Geometry check sheet. Reference: the model listing, model coordinates, mm. A direction names the side the tool comes from. Give positions to 0.01 mm unless a question says otherwise; leave off trailing zeros. Order: outer loops, then holes, each group sorted by start corner. A loop starts at its lowest first (then second) coordinate and runs counter-clockwise, first axis right, second up. Notation, with made-up numbers: M 71,78 L 79,78 A35 ccw 79,115 Z; hole C 18,8.25 d6. An arc over 180 degrees is marked long. Answer as a JSON object with one key per item and string values. Group by question number.
from build123d import *

# Parameters (mm, degrees)
F1_DEPTH     = 2
F3_DEPTH     = 13
F4_DEPTH     = 11
F5_R         = 1.5
F6_DEPTH     = 8
F7_T4_DEPTH  = 97.0812194284
F7_T9_DEPTH  = 97.0812194284
F7_T14_DEPTH = 97.0812194284
F7_T20_DEPTH = 97.0812194284
F7_T25_DEPTH = 97.0812194284
F7_T31_DEPTH = 97.0812194284
F8_R         = 1


# Not quite as in the source:
# - a fillet or chamfer that OpenCascade refuses, or shapes differently, is made with other operations: its cross-section is extruded or revolved along the edge and cut away or added


with BuildPart() as f1:
    # F0 (on Top) → F1 (new body)
    with BuildSketch(Plane.XY):
        Polygon((0, 9.3), (0, 0), (67, 0), (67, 6), align=None)
    extrude(amount=F1_DEPTH)

    # F2 (on face) → F3 (join)
    with BuildSketch(Plane.XY.offset(2)):
        Polygon((0.7854075007, 8.5), (0.7854075007, 0.5), (8.7757214003, 8.1064472258), align=None)
    extrude(amount=-F3_DEPTH)

    # F2 (on face) → F4 (join)
    with BuildSketch(Plane.XY.offset(2)):
        Polygon((62.9, 1.65), (66.9, 5.8), (53.9157399132, 6.439523258), (57.3, 1.65), align=None)
    extrude(amount=-F4_DEPTH)

    # F5 (on face) → F6 (cut)
    with BuildSketch(Plane(origin=(0, 0, -11), x_dir=(1, 0, 0), z_dir=(0, 0, -1))):
        with Locations((3.1854075007, -5.9788816921)):
            Circle(F5_R)
        with Locations((60.0157399132, -3.9364085902)):
            Circle(F5_R)
    extrude(amount=-F6_DEPTH, mode=Mode.SUBTRACT)

    # F7: fillet of radius 10 on 1 edges, made by hand


with BuildPart() as f7_tool2:
    # F7_s3 → F7_t4 (new body)
    with BuildSketch(Plane(origin=(81.5248873918, -4.0154049014, 0), x_dir=(0, 0, 1), z_dir=(-0.9987892374, 0.0491940968, 0))):
        with BuildLine():
            ThreePointArc((2, 9.2887399083), (0.5131670195, 6.4510175684), (0, 3.2887399083))
            Line((0, 3.2887399083), (0, 9.2887399083))
            Line((0, 9.2887399083), (2, 9.2887399083))
        make_face()
    extrude(amount=F7_T4_DEPTH)

    split(bisect_by=Plane(origin=(0.4468822571, 9.0730640082, 0), x_dir=(0, 0, 1), z_dir=(0.0491940968, 0.9987892374, 0)), keep=Keep.TOP)


with BuildPart() as f1_1:
    add(f1.part)

    # F7_t1: cut F7_tool2
    add(f7_tool2.part, mode=Mode.SUBTRACT)


with BuildPart() as f7_tool7:
    # F7_s8 → F7_t9 (new body)
    with BuildSketch(Plane(origin=(81.5248873918, -4.0154049014, 0), x_dir=(0, 0, 1), z_dir=(-0.9987892374, 0.0491940968, 0))):
        with BuildLine():
            ThreePointArc((2, 9.2887399083), (0.5131670195, 6.4510175684), (0, 3.2887399083))
            Line((0, 3.2887399083), (0, 9.2887399083))
            Line((0, 9.2887399083), (2, 9.2887399083))
        make_face()
    extrude(amount=F7_T9_DEPTH)

    split(bisect_by=Plane(origin=(31.7828354278, -30.6340582437, 0), x_dir=(0, 0, 1), z_dir=(0.7199990803, -0.6939750171, 0)), keep=Keep.TOP)


with BuildPart() as f1_2:
    add(f1_1.part)

    # F7_t6: cut F7_tool7
    add(f7_tool7.part, mode=Mode.SUBTRACT)


with BuildPart() as f7_tool12:
    # F7_s13 → F7_t14 (new body)
    with BuildSketch(Plane(origin=(81.5248873918, -4.0154049014, 0), x_dir=(0, 0, 1), z_dir=(-0.9987892374, 0.0491940968, 0))):
        with BuildLine():
            ThreePointArc((2, 9.2887399083), (0.5131670195, 6.4510175684), (0, 3.2887399083))
            Line((0, 3.2887399083), (0, 9.2887399083))
            Line((0, 9.2887399083), (2, 9.2887399083))
        make_face()
    extrude(amount=F7_T14_DEPTH)

    split(bisect_by=Plane(origin=(38.996012386, 27.554443554, 0), x_dir=(0, 0, 1), z_dir=(-0.816693011, -0.5770723748, 0)), keep=Keep.TOP)

    split(bisect_by=Plane(origin=(0.1236877347, -0.1299297552, 0), x_dir=(0, 0, 1), z_dir=(0.6894947075, -0.7242907209, 0)), keep=Keep.TOP)


with BuildPart() as f1_3:
    add(f1_2.part)

    # F7_t11: cut F7_tool12
    add(f7_tool12.part, mode=Mode.SUBTRACT)


with BuildPart() as f7_tool18:
    # F7_s19 → F7_t20 (new body)
    with BuildSketch(Plane(origin=(81.5248873918, -4.0154049014, 0), x_dir=(0, 0, 1), z_dir=(-0.9987892374, 0.0491940968, 0))):
        with BuildLine():
            ThreePointArc((2, 9.2887399083), (0.5131670195, 6.4510175684), (0, 3.2887399083))
            Line((0, 3.2887399083), (0, 9.2887399083))
            Line((0, 9.2887399083), (2, 9.2887399083))
        make_face()
    extrude(amount=F7_T20_DEPTH)

    split(bisect_by=Plane.XZ.offset(-1.65), keep=Keep.TOP)


with BuildPart() as f1_4:
    add(f1_3.part)

    # F7_t17: cut F7_tool18
    add(f7_tool18.part, mode=Mode.SUBTRACT)


with BuildPart() as f7_tool23:
    # F7_s24 → F7_t25 (new body)
    with BuildSketch(Plane(origin=(81.5248873918, -4.0154049014, 0), x_dir=(0, 0, 1), z_dir=(-0.9987892374, 0.0491940968, 0))):
        with BuildLine():
            ThreePointArc((2, 9.2887399083), (0.5131670195, 6.4510175684), (0, 3.2887399083))
            Line((0, 3.2887399083), (0, 9.2887399083))
            Line((0, 9.2887399083), (2, 9.2887399083))
        make_face()
    extrude(amount=F7_T25_DEPTH)

    split(bisect_by=Plane(origin=(0.419544275, 8.518020129, 0), x_dir=(0, 0, 1), z_dir=(0.0491940968, 0.9987892374, 0)), keep=Keep.TOP)

    split(bisect_by=Plane(origin=(0.1236877347, -0.1299297552, 0), x_dir=(0, 0, 1), z_dir=(-0.6894947075, 0.7242907209, 0)), keep=Keep.TOP)


with BuildPart() as f1_5:
    add(f1_4.part)

    # F7_t22: cut F7_tool23
    add(f7_tool23.part, mode=Mode.SUBTRACT)


with BuildPart() as f7_tool29:
    # F7_s30 → F7_t31 (new body)
    with BuildSketch(Plane(origin=(81.5248873918, -4.0154049014, 0), x_dir=(0, 0, 1), z_dir=(-0.9987892374, 0.0491940968, 0))):
        with BuildLine():
            ThreePointArc((2, 9.2887399083), (0.5131670195, 6.4510175684), (0, 3.2887399083))
            Line((0, 3.2887399083), (0, 9.2887399083))
            Line((0, 9.2887399083), (2, 9.2887399083))
        make_face()
    extrude(amount=F7_T31_DEPTH)

    split(bisect_by=Plane.YZ.offset(0.7854075007), keep=Keep.BOTTOM)


with BuildPart() as f1_6:
    add(f1_5.part)

    # F7_t28: cut F7_tool29
    add(f7_tool29.part, mode=Mode.SUBTRACT)

    # F8
    f8_edges = [f1_6.edges().sort_by_distance(p)[0] for p in [
        (0.785408, 8.5, -4.758713),
        (8.775721, 8.106447, -4.758713),
        (0.785408, 0.5, -5.5),
        (66.9, 5.8, -3.574746),
        (53.91574, 6.439523, -3.574746),
    ]]
    fillet(f8_edges, radius=F8_R)

    # F9: F1 across plane


with BuildPart() as f1_7:
    add(f1_6.part)
    add(f1_6.part.mirror(Plane.XZ))


solid = f1_7.part
1. Thickness scan on line 1 along Z through (x, y) = (23.5, 2.5); line 2 along X through (y, z) = (6.5, -2.5); line 3 along Y through (x, z) = (4, -7.75). Record the ranges inside material, lowest first. Write a range as [from, to].
2. Release check for a two-part mould opening along X. For faces 1 (the flat face through (3, 4, -11)), 2 (the flat face through (3, 6, -3)), 3 (the flat face through (67, 0, 1)) record: released by +X, released by -X, zero draft, split by the parting line, or undercut.
3. Cross-section at B-B (z = -5.25). Record the cut outline in (x, y), and give its area (3 significant figures).
4. Cross-section at A-A (z = -2.25). Record the cut outline in (x, y), and give its area (3 significant figures).
5. Access from +Z, -Z, +X, -X, +Y, -Y to the whole of each face (thin tool, end or side, straight path). Record for faces 4 (the flat face through (60, 4, -3)), 5 (the flat face through (60.2, -5.6, -9)), 6 (the flat face through (0, 0, 1)).
6. Depth check by flat-ended pin: pin 1 (1.4 mm diameter, centred on x = 62, y = -3.5, fed in from -Z); pin 2 (3.5 mm diameter, centred on y = -6, z = -6, fed in from -X); pin 3 (0.9 mm diameter, centred on x = 3.5, y = 6, fed in from -Z). Enter the tip coordinate at first touch or a pass-through.
Report:
{
 "1": {"line 1": "z = [0.01, 2]", "line 2": "x = [0.79, 7.09]", "line 3": "y = [-8.34, -7.24], [-4.72, -3.56], [3.56, 4.72], [7.24, 8.34]"},
 "2": {"face 1": "zero draft", "face 2": "undercut", "face 3": "released by +X"},
 "3": {"outline": "M 0.79,-7.45 A1 ccw 1.83,-8.45 L 6.45,-8.22 A1 ccw 7.09,-6.5 L 2.47,-2.11 A1 ccw 0.79,-2.83 Z; M 0.79,2.83 A1 ccw 2.47,2.11 L 7.09,6.5 A1 ccw 6.45,8.22 L 1.83,8.45 A1 ccw 0.79,7.45 Z; M 55.1,-4.76 A1 ccw 55.97,-6.34 L 64.7,-5.91 A1 ccw 65.37,-4.22 L 62.9,-1.65 L 57.3,-1.65 Z; M 55.1,4.76 L 57.3,1.65 L 62.9,1.65 L 65.37,4.22 A1 ccw 64.7,5.91 L 55.97,6.34 A1 ccw Z; hole C 3.19,-5.98 d3; hole C 3.19,5.98 d3; hole C 60.02,-3.94 d3; hole C 60.02,3.94 d3", "area": "110 mm2"},
 "4": {"outline": "M 0.79,-7.45 A1 ccw 1.83,-8.45 L 6.45,-8.22 A1 ccw 7.09,-6.5 L 2.47,-2.11 A1 ccw 0.79,-2.83 Z; M 0.79,2.83 A1 ccw 2.47,2.11 L 7.09,6.5 A1 ccw 6.45,8.22 L 1.83,8.45 A1 ccw 0.79,7.45 Z; M 55.1,-4.76 A1 ccw 55.97,-6.34 L 64.7,-5.91 A1 ccw 65.37,-4.22 L 62.9,-1.65 L 57.3,-1.65 Z; M 55.1,4.76 L 57.3,1.65 L 62.9,1.65 L 65.37,4.22 A1 ccw 64.7,5.91 L 55.97,6.34 A1 ccw Z", "area": "138 mm2"},
 "5": {"face 4": "-Z", "face 5": "-Z, +X, +Y, -Y", "face 6": "+Z, -Z, -X, +Y, -Y"},
 "6": {"pin 1": "stops at z = -9", "pin 2": "stops at x = 0.79", "pin 3": "stops at z = -3"}
}
